from build123d import *

# Parameters (mm, degrees)
F0_W     = 1270
F0_H     = 508
F1_DEPTH = 25.4
F2_W     = 127
F2_H     = 508
F3_DEPTH = 390.525
F5_DEPTH = 1270.001


with BuildPart() as f1:
    # F0 (on Top) → F1 (new body)
    with BuildSketch(Plane.XY):
        Rectangle(F0_W, F0_H)
    extrude(amount=F1_DEPTH)

    # F2 (on face) → F3 (join)
    with BuildSketch(Plane(origin=(0, 0, 0), x_dir=(1, 0, 0), z_dir=(0, 0, -1))):
        with Locations((-571.5, 0)):
            Rectangle(F2_W, F2_H)
        with Locations((571.5, 0)):
            Rectangle(F2_W, F2_H)
    extrude(amount=F3_DEPTH)

    # F4 (on face) → F5 (cut, through all)
    with BuildSketch(Plane.YZ.offset(635)):
        Polygon((0, -243.319523), (-141.925823, -352.425), (141.925823, -352.425), align=None)
        Polygon((215.9, -77.346398), (62.513201, -195.2625), (215.9, -313.178602), align=None)
        Polygon((0, -147.205477), (141.925823, -38.1), (-141.925823, -38.1), align=None)
        Polygon((-215.9, -313.178602), (-62.513201, -195.2625), (-215.9, -77.346398), align=None)
    extrude(amount=-F5_DEPTH, mode=Mode.SUBTRACT)


solid = f1.part
Model file for the job. Use its own axes, mm. A direction names the side the tool comes from. Round coordinates to 2 decimals unless told otherwise and drop trailing zeros. Order: outer loops, then holes, each group sorted by start corner. A loop starts at its lowest first (then second) coordinate and runs counter-clockwise, first axis right, second up.
(1) Band-saw the part on A-A (y = -170). List the corners of the cut face in (x, z) (3 decimals), then the cut area to 3 significant figures.
(2) Band-saw the part on D-D (z = -64.5). List the corners of the cut face in (x, y).
(3) Pin check, flat tip, straight feed: pin 1 (6 mm diameter, centred on x = 268.5, y = 50.5, fed in from -Z). Stop position of the tip, or through.
(4) Drill centre lines: line 1 (X direction, y = -145, z = -351.5); line 2 (Z direction, x = -515.5, y = -89.5) (3 decimals); line 3 (Z direction, x = -227, y = 209). Where is each one in solid material? Low to high.
(5) 3-axis set-ups, long thin cutter, end or side, ignore diameter. For faces 1 (the face through (-570.611, 138.133, -253.395)), 2 (the face through (-635, 4, -180)): which of +Z, -Z, +X, -X, +Y, -Y reach the whole face in a straight line?
(6) Band-saw the part on C-C (y = -30.5). List the corners of the cut face in (x, z) (3 decimals).
(7) Band-saw the part on B-B (z = -275). Give the number of separate pieces and of enclosed holes in the cut face, then the cut area to 3 significant figures.
(8) Pull direction Y, two halves, no side cores. Call faces 3 (the face through (508, 4, -193)), 4 (the face through (-3, 254, 19)), 5 (the face through (572.389, 69.969, -93.416)): released by +Y, released by -Y, zero draft, split by the parting line, or undercut.
Verdict:
1. outline: (-635, -390.525) - (-508, -390.525) - (-508, -277.893) - (-635, -277.893) - close; (-635, -112.632) - (-508, -112.632) - (-508, 0) - (508, 0) - (508, -112.632) - (635, -112.632) - (635, 25.4) - (-635, 25.4) - close; (508, -390.525) - (635, -390.525) - (635, -277.893) - (508, -277.893) - close
1. area: 89,500 mm2
2. outline: (-635, -254) - (-508, -254) - (-508, -107.58) - (-635, -107.58) - close; (-635, 107.58) - (-508, 107.58) - (-508, 254) - (-635, 254) - close; (508, -254) - (635, -254) - (635, -107.58) - (508, -107.58) - close; (508, 107.58) - (635, 107.58) - (635, 254) - (508, 254) - close
3. pin 1: stops at z = 0
4. line 1: x = -635 to -508, 508 to 635
4. line 2: z = -390.525 to -352.425, -312.123 to -216.009, -174.516 to -78.402, -38.1 to 25.4
4. line 3: z = 0 to 25.4
5. face 1: +X, -X
5. face 2: +Z, -Z, -X, +Y, -Y
6. outline: (-635, -390.525) - (-508, -390.525) - (-508, -352.425) - (-635, -352.425) - close; (-635, -266.766) - (-508, -266.766) - (-508, -123.759) - (-635, -123.759) - close; (-635, -38.1) - (-508, -38.1) - (-508, 0) - (508, 0) - (508, -38.1) - (635, -38.1) - (635, 25.4) - (-635, 25.4) - close; (508, -390.525) - (635, -390.525) - (635, -352.425) - (508, -352.425) - close; (508, -266.766) - (635, -266.766) - (635, -123.759) - (508, -123.759) - close
7. separate pieces: 8
7. enclosed holes: 0
7. area: 82,900 mm2
8. face 3: zero draft
8. face 4: released by +Y
8. face 5: undercut
